For this review, use the dimensioned drawing (mm, ordinates from the lowest corner) and the shaded views. A direction names the side the tool comes from. Coordinates: 2 decimals unless noted, no trailing zeros. Write each loop counter-clockwise with the first axis right and the second up, starting at its lowest first coordinate (ties: lowest second). Pieces come first, ordered by that corner, then holes. Notation, with made-up numbers: (21, 25.25) -> (55, 25.25) arc R16 cw to (55, 33.25) -> close; hole circle Ø9 at (-37, 19). An arc over 180 degrees is marked (long way). Put each result on its own line as item: value. Start each with the question number.
Item 1: Consider section C-C on x = 4. Give the boundary of the cut face in (y, z), and give its area (3 significant figures).
Item 2: For the marked faces 1, 2 and 3, list the 3-axis set-ups (+Z, -Z, +X, -X, +Y, -Y) from which the entire face can be reached by the end or side of a thin tool; tool diameter is ignored.
Item 3: The part is to be moulded in two halves that separate along Y. For the marked faces 4, 5, 6 and 7, say which applies: +Y half, -Y half, draft (parallel to the pull), parting line (faces both ways), or undercut.
Item 4: Consider section B-B on y = 8. Give the boundary of the cut face in (x, z).
Item 5: Insertion check: P1, Ø0.8, axis at x = 4, y = 12, coming from the -Z side; P2, Ø1.5, axis at y = 8.5, z = 7, coming from the -X side. Each pin has a flat end and moves straight along its axis. Give the tip position at first contact, or say it passes through.
Item 6: To check wall thickness, follow L1, parallel to Y at x = 12, z = 8.75; L2, parallel to Y at x = 8, z = 5.5. State the ranges of each line that lie inside material, in increasing order.
Item 7: Consider section A-A on z = 1.25. Give the boundary of the cut face in (x, y), and give its area (3 significant figures).
Item 8: Consider section D-D on z = 10.25. Give the boundary of the cut face in (x, y), and give its area (3 significant figures).
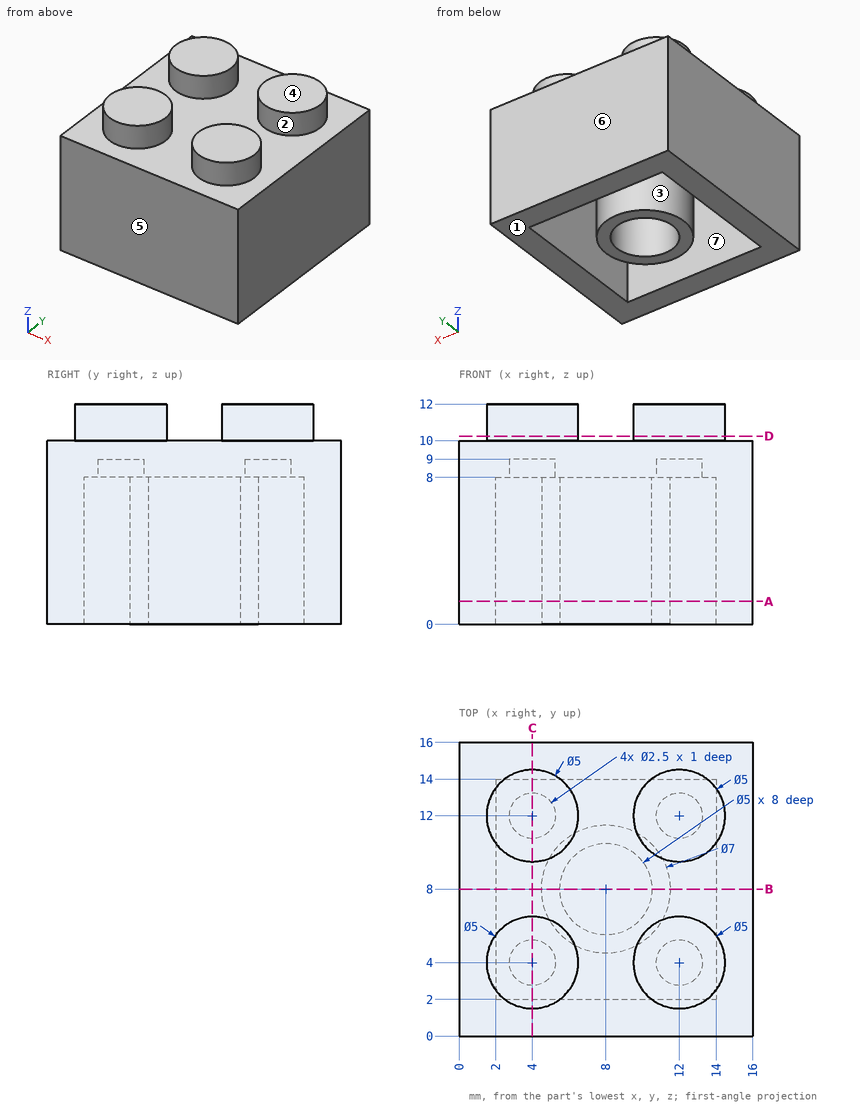
Return value:
1. outline: (0, 0) -> (2, 0) -> (2, 8) -> (2.75, 8) -> (2.75, 9) -> (5.25, 9) -> (5.25, 8) -> (10.75, 8) -> (10.75, 9) -> (13.25, 9) -> (13.25, 8) -> (14, 8) -> (14, 0) -> (16, 0) -> (16, 10) -> (14.5, 10) -> (14.5, 12) -> (9.5, 12) -> (9.5, 10) -> (6.5, 10) -> (6.5, 12) -> (1.5, 12) -> (1.5, 10) -> (0, 10) -> close
1. area: 79.0 mm^2
2. face 1: -Z, +X, -X, +Y, -Y
2. face 2: +Z
2. face 3: -Z
3. face 4: draft
3. face 5: -Y half
3. face 6: +Y half
3. face 7: undercut
4. outline: (0, 0) -> (2, 0) -> (2, 8) -> (4.5, 8) -> (4.5, 0) -> (5.5, 0) -> (5.5, 8) -> (10.5, 8) -> (10.5, 0) -> (11.5, 0) -> (11.5, 8) -> (14, 8) -> (14, 0) -> (16, 0) -> (16, 10) -> (0, 10) -> close
5. P1: z = 9
5. P2: x = 0
6. L1: 0 to 2.75, 5.25 to 10.75, 13.25 to 16
6. L2: 0 to 2, 4.5 to 5.5, 10.5 to 11.5, 14 to 16
7. outline: (0, 0) -> (16, 0) -> (16, 16) -> (0, 16) -> close; circle Ø7 at (8, 8); hole (2, 2) -> (14, 2) -> (14, 14) -> (2, 14) -> close; hole circle Ø5 at (8, 8)
7. area: 131 mm^2
8. outline: circle Ø5 at (4, 4); circle Ø5 at (4, 12); circle Ø5 at (12, 4); circle Ø5 at (12, 12)
8. area: 78.5 mm^2
